```python
from build123d import *

# Parameters (mm, degrees)
SKETCH1_R           = 2
BOSS_EXTRUDE1_DEPTH = 4
BOSS_EXTRUDE2_DEPTH = 16.4
SKETCH3_R           = 3
BOSS_EXTRUDE3_DEPTH = 3
FILLET1_R           = 10
BOSS_EXTRUDE4_DEPTH = 10
FILLET3_R           = 10
CUT_EXTRUDE3_DEPTH  = 7.5
SKETCH9_W           = 25
SKETCH9_H           = 14
CUT_EXTRUDE4_DEPTH  = 15
FILLET4_R           = 20
SKETCH10_R          = 2.55
CUT_EXTRUDE5_DEPTH  = 4


with BuildPart() as part:
    # Sketch1 → Boss-Extrude1 (new body)
    with BuildSketch(Plane.XY):
        with BuildLine():
            Line((80, -25), (-80, -25))
            ThreePointArc((-80, -25), (-105, 0), (-80, 25))
            Line((-80, 25), (80, 25))
            ThreePointArc((80, 25), (105, 0), (80, -25))
        make_face()
        with Locations((75, -15)):
            Circle(SKETCH1_R, mode=Mode.SUBTRACT)
        with Locations((75, 15)):
            Circle(SKETCH1_R, mode=Mode.SUBTRACT)
        with Locations((-75, -15)):
            Circle(SKETCH1_R, mode=Mode.SUBTRACT)
        with Locations((-75, 15)):
            Circle(SKETCH1_R, mode=Mode.SUBTRACT)
        with BuildLine():
            Line((47.5, -14.5), (-47.5, -14.5))
            ThreePointArc((-47.5, -14.5), (-62, 0), (-47.5, 14.5))
            Line((-47.5, 14.5), (47.5, 14.5))
            ThreePointArc((47.5, 14.5), (62, 0), (47.5, -14.5))
        make_face(mode=Mode.SUBTRACT)
    extrude(amount=BOSS_EXTRUDE1_DEPTH)

    # Sketch2 → Boss-Extrude2 (add)
    with BuildSketch(Plane.XY.offset(4)):
        with BuildLine():
            Line((80, 25), (-80, 25))
            ThreePointArc((-80, 25), (-105, 0), (-80, -25))
            Line((-80, -25), (80, -25))
            ThreePointArc((80, -25), (105, 0), (80, 25))
        make_face()
        with BuildLine():
            Line((47.5, 14.5), (-47.5, 14.5))
            ThreePointArc((-47.5, 14.5), (-62, 0), (-47.5, -14.5))
            Line((-47.5, -14.5), (47.5, -14.5))
            ThreePointArc((47.5, -14.5), (62, 0), (47.5, 14.5))
        make_face(mode=Mode.SUBTRACT)
    extrude(amount=BOSS_EXTRUDE2_DEPTH)

    # Sketch3 → Boss-Extrude3 (add)
    with BuildSketch(Plane.XY.offset(20.4)):
        with BuildLine():
            Line((80, 25), (-80, 25))
            ThreePointArc((-80, 25), (-105, 0), (-80, -25))
            Line((-80, -25), (80, -25))
            ThreePointArc((80, -25), (105, 0), (80, 25))
        make_face()
        with Locations((-47.5, 0)):
            Circle(SKETCH3_R, mode=Mode.SUBTRACT)
        with Locations((47.5, 0)):
            Circle(SKETCH3_R, mode=Mode.SUBTRACT)
    extrude(amount=BOSS_EXTRUDE3_DEPTH)

    # Fillet1
    fillet1_edges = [part.edges().sort_by_distance(p)[0] for p in [
        (105, 0, 23.4),
        (0, 25, 23.4),
        (-105, 0, 23.4),
        (0, -25, 23.4),
    ]]
    fillet(fillet1_edges, radius=FILLET1_R)

    # Sketch4 → Boss-Extrude4 (add)
    with BuildSketch(Plane(origin=(0, 0, 0), x_dir=(-1, 0, 0), z_dir=(0, 0, -1))):
        with BuildLine():
            Line((80, 25), (105, 55.206564225))
            ThreePointArc((105, 55.206564225), (113.254710442, 27.603282112), (105, 0))
            ThreePointArc((105, 0), (97.67766953, 17.67766953), (80, 25))
        make_face()
        with BuildLine():
            Line((-80, 25), (-105, 55.206564225))
            ThreePointArc((-105, 55.206564225), (-113.254710442, 27.603282112), (-105, 0))
            ThreePointArc((-105, 0), (-97.67766953, 17.67766953), (-80, 25))
        make_face()
    extrude(amount=-BOSS_EXTRUDE4_DEPTH)

    # Fillet3
    fillet3_edges = [part.edges().sort_by_distance(p)[0] for p in [
        (105, 55.206564225, 5),
        (-105, 55.206564225, 5),
    ]]
    fillet(fillet3_edges, radius=FILLET3_R)

    # Sketch8 → Cut-Extrude3 (cut)
    with BuildSketch(Plane(origin=(0, 0, 0), x_dir=(-1, 0, 0), z_dir=(0, 0, -1))):
        with BuildLine():
            Line((-100.820886267, 2.744996978), (-83.851879902, 21.812050625))
            Line((-83.851879902, 21.812050625), (-98.458728042, 39.460958483))
            ThreePointArc((-98.458728042, 39.460958483), (-103.485584806, 41.132991554), (-107.19341332, 37.349211536))
            ThreePointArc((-107.19341332, 37.349211536), (-107.505926341, 19.402788283), (-100.820886267, 2.744996978))
        make_face()
        with BuildLine():
            Line((83.851879902, 21.812050625), (98.458728042, 39.460958483))
            ThreePointArc((98.458728042, 39.460958483), (103.485584806, 41.132991554), (107.19341332, 37.349211536))
            ThreePointArc((107.19341332, 37.349211536), (107.505926341, 19.402788283), (100.820886267, 2.744996978))
            Line((100.820886267, 2.744996978), (83.851879902, 21.812050625))
        make_face()
    extrude(amount=-CUT_EXTRUDE3_DEPTH, mode=Mode.SUBTRACT)

    # Sketch9 → Cut-Extrude4 (cut)
    with BuildSketch(Plane.XZ.offset(25)):
        with Locations((40, 13.4)):
            Rectangle(SKETCH9_W, SKETCH9_H)
    extrude(amount=-CUT_EXTRUDE4_DEPTH, mode=Mode.SUBTRACT)

    # Fillet4
    # the kernel refuses this fillet: 20 mm, written as the material it adds along each edge
    with BuildSketch(Plane(origin=(80, 25, 10), x_dir=(-1, 0, 0), z_dir=(0, 0, -1)), Plane(origin=(-80, 25, 10), x_dir=(-0.6375898750759507, 0.7703759804151696, 0), z_dir=(0, 0, -1))) as fillet4_piece_1:
        with BuildLine():
            CenterArc((FILLET4_R * 0.470432794035, FILLET4_R), FILLET4_R, 219.612336421, 50.387663579)
            Line((-FILLET4_R * 0.29994318638, FILLET4_R * 0.362410124924), (0, 0))
            Line((0, 0), (FILLET4_R * 0.470432794035, 0))
        make_face()
    extrude(amount=10)

    # Sketch10 → Cut-Extrude5 (cut)
    with BuildSketch(Plane.XZ.offset(25)):
        with Locations((-5, 6.7)):
            Circle(SKETCH10_R)
        with Locations(Location((5, 6.7, 0), (0, 0, 180))):
            Circle(SKETCH10_R)
    extrude(amount=-CUT_EXTRUDE5_DEPTH, mode=Mode.SUBTRACT)


solid = part.part
```
Geometry check sheet. Reference: the model listing, model coordinates, mm. A direction names the side the tool comes from. Give positions to 0.01 mm unless a question says otherwise; leave off trailing zeros. Write each loop counter-clockwise with the first axis right and the second up, starting at its lowest first coordinate (ties: lowest second). Pieces come first, ordered by that corner, then holes.
1) Gauge pin test, flat ends, axial feed: pin 1 (3 mm diameter, centred on x = 5, z = 6.7, fed in from -Y); pin 2 (11.5 mm diameter, centred on y = -17.5, z = 13, fed in from +X); pin 3 (10 mm diameter, centred on x = -90, z = 6, fed in from +Y); pin 4 (10 mm diameter, centred on x = -78, y = 32, fed in from -Z). Record the tip position at first contact, or that the pin passes through.
2) Section check A-A, the plane x = 42.5. Record the boundary of the cut face in (y, z), and give its area (3 significant figures).
3) Release check for a two-part mould opening along Y. For faces 6 (the flat face through (40, -19, 6.4)), 7 (the flat face through (1, 14.5, 10)), 8 (the flat face through (75, 15, 4)), 9 (the flat face through (1, 25, 7)) record: pulls with the +Y half, pulls with the -Y half, needs draft (parallel to the pull), parting line crosses it, or undercut.
4) Access from +Z, -Z, +X, -X, +Y, -Y to the whole of each face (thin tool, end or side, straight path). Record for faces 1 (the cylindrical face through (-1.12, 21.99, 20.55)), 2 (the cylindrical face through (-104.51, 46.03, 5.07)), 3 (the cylindrical face through (-2.57, -23.03, 7.47)), 4 (the flat face through (91.05, 30.51, 3.7)), 5 (the flat face through (-99, 27, 10)).
5) Section check D-D, the plane x = -59. Record the boundary of the cut face in (y, z).
6) Material ranges on L1, parallel to X at y = 40, z = 5.5; L2, parallel to Y at x = 10, z = 5.5; L3, parallel to Z at x = -11.5, y = 11, recorded low to high.
7) Section check C-C, the plane z = 15.75. Record the boundary of the cut face in (x, y), and give its area (3 significant figures).
8) Section check B-B, the plane x = -5. Record the boundary of the cut face in (y, z).
Computed:
1. pin 1: stops at y = -21
1. pin 2: stops at x = 102.07
1. pin 3: stops at y = 43.1
1. pin 4: passes through
2. outline: (-25, 0) - (-14.5, 0) - (-14.5, 6.4) - (-25, 6.4) - close; (-22.14, 20.4) - (14.5, 20.4) - (14.5, 0) - (25, 0) - (25, 13.4) arc R10 ccw to (15, 23.4) - (-15, 23.4) arc R10 ccw to start
2. area: 395 mm2
3. face 6: needs draft
3. face 7: undercut
3. face 8: undercut
3. face 9: pulls with the +Y half
4. face 1: +Z, +X, -X, +Y
4. face 2: +Z, -Z, +Y
4. face 3: -Y
4. face 4: -Z
4. face 5: +Z, -X, +Y
5. outline: (-25, 0) - (-8.83, 0) - (-8.83, 20.4) - (8.83, 20.4) - (8.83, 0) - (25, 0) - (25, 13.4) arc R10 ccw to (15, 23.4) - (-15, 23.4) arc R10 ccw to (-25, 13.4) - close
6. L1: x = -111.59 to -105.64, -98.98 to -92.41, 92.41 to 98.98, 105.64 to 111.59
6. L2: y = -25 to -14.5, 14.5 to 25
6. L3: z = 20.4 to 23.4
7. outline: (-80, -24.72) - (27.5, -24.72) - (27.5, -14.5) - (-47.5, -14.5) arc R14.5 cw to (-47.5, 14.5) - (47.5, 14.5) arc R14.5 cw to (52.5, -13.61) - (52.5, -24.72) - (80, -24.72) arc R24.72 ccw to (80, 24.72) - (-80, 24.72) arc R24.72 ccw to start
7. area: 6,160 mm2
8. outline: (-25, 0) - (-14.5, 0) - (-14.5, 20.4) - (14.5, 20.4) - (14.5, 0) - (25, 0) - (25, 13.4) arc R10 ccw to (15, 23.4) - (-15, 23.4) arc R10 ccw to (-25, 13.4) - (-25, 9.25) - (-21, 9.25) - (-21, 4.15) - (-25, 4.15) - close
